Verification items for the finished model (mm, model axes). A direction names the side the tool comes from. Round coordinates to 2 decimals unless told otherwise and drop trailing zeros. Write each loop counter-clockwise with the first axis right and the second up, starting at its lowest first coordinate (ties: lowest second). Pieces come first, ordered by that corner, then holes. Notation, with made-up numbers: (62.25, 83.25) - (67.25, 83.25) arc R15 cw to (67.25, 105.25) - close; hole circle Ø11 at (12.25, -8). An arc over 180 degrees is marked (long way). Answer as a JSON object with one key per item and string values.
```python
from build123d import *

# Parameters (mm, degrees)
SKETCH1_W                        = 80
SKETCH1_H                        = 140
SKETCH1_R                        = 12.5
BOSS_EXTRUDE1_DEPTH              = 6
TAP_DRILL_FOR_M6_TAP1_D          = 5
TAP_DRILL_FOR_M6_TAP2_AT_2_COUNT = 2
TAP_DRILL_FOR_M6_TAP2_AT_2_PITCH = 32.5
TAP_DRILL_FOR_M6_TAP2_AT_3_COUNT = 2
TAP_DRILL_FOR_M6_TAP2_AT_3_PITCH = 65
TAP_DRILL_FOR_M6_TAP3_D          = 5
TAP_DRILL_FOR_M6_TAP3_DEPTH      = 26
TAP_DRILL_FOR_M6_TAP3_TIP        = 1.502151548


with BuildPart() as part:
    # Sketch1 → Boss-Extrude1 (new body, symmetric)
    with BuildSketch(Plane(origin=(0, 0, 0), x_dir=(1, 0, 0), z_dir=(0, 1, 0))):
        with Locations((0, 70)):
            Rectangle(SKETCH1_W, SKETCH1_H)
        with Locations((10, 42.5)):
            Circle(SKETCH1_R, mode=Mode.SUBTRACT)
    extrude(amount=BOSS_EXTRUDE1_DEPTH, both=True)

    # Tap Drill for M6 Tap1 (through all)
    with Locations(Plane(origin=(0, 6, 0), x_dir=(1, 0, 0), z_dir=(0, 1, 0))):
        with Locations((-25, 67.5), (25, 67.5), (25, 17.5), (-25, 17.5)):
            Hole(TAP_DRILL_FOR_M6_TAP1_D / 2)

    # Sketch9 → Tap Drill for M6 Tap2 (revolve, cut)
    with BuildSketch(Plane(origin=(32.5, 0, 0), x_dir=(0, -1, 0), z_dir=(1, 0, 0))):
        Polygon((0, 0), (0, 21.502151548), (2.5, 20), (2.5, 0), align=None)
    tap_drill_for_m6_tap2 = revolve(axis=Axis((32.5, 0, 6.35), (0, 0, -1)), mode=Mode.SUBTRACT)

    # Tap Drill for M6 Tap2 at 2: Tap Drill for M6 Tap2 ×2
    with Locations(*[(-i * TAP_DRILL_FOR_M6_TAP2_AT_2_PITCH, 0, 0) for i in range(1, TAP_DRILL_FOR_M6_TAP2_AT_2_COUNT)]):
        add(tap_drill_for_m6_tap2, mode=Mode.SUBTRACT)

    # Tap Drill for M6 Tap2 at 3: Tap Drill for M6 Tap2 ×2
    with Locations(*[(-i * TAP_DRILL_FOR_M6_TAP2_AT_3_PITCH, 0, 0) for i in range(1, TAP_DRILL_FOR_M6_TAP2_AT_3_COUNT)]):
        add(tap_drill_for_m6_tap2, mode=Mode.SUBTRACT)

    # Mirror1: Tap Drill for M6 Tap2 across plane
    add(tap_drill_for_m6_tap2.mirror(Plane(origin=(0, 0, -70), x_dir=(1, 0, 0), z_dir=(0, 0, -1))), mode=Mode.SUBTRACT)

    # Mirror1 copy 1 sketch → Mirror1 copy 1 (revolve, cut)
    with BuildSketch(Plane(origin=(0, 0, -140), x_dir=(0, -1, 0), z_dir=(1, 0, 0))):
        Polygon((0, 0), (0, -21.502151548), (2.5, -20), (2.5, 0), align=None)
    revolve(axis=Axis((0, 0, -146.35), (0, 0, -1)), mode=Mode.SUBTRACT)

    # Mirror1 copy 2 sketch → Mirror1 copy 2 (revolve, cut)
    with BuildSketch(Plane(origin=(-32.5, 0, -140), x_dir=(0, -1, 0), z_dir=(1, 0, 0))):
        Polygon((0, 0), (0, -21.502151548), (2.5, -20), (2.5, 0), align=None)
    revolve(axis=Axis((-32.5, 0, -146.35), (0, 0, -1)), mode=Mode.SUBTRACT)

    # Tap Drill for M6 Tap3
    with Locations(Plane.ZY.offset(40)):
        with Locations((-113, 0), (-86, 0), (-56, 0), (-29, 0)):
            Hole(TAP_DRILL_FOR_M6_TAP3_D / 2, depth=TAP_DRILL_FOR_M6_TAP3_DEPTH)
            with Locations((0, 0, -(TAP_DRILL_FOR_M6_TAP3_DEPTH + TAP_DRILL_FOR_M6_TAP3_TIP / 2))):  # 118° drill point
                Cone(0, TAP_DRILL_FOR_M6_TAP3_D / 2, TAP_DRILL_FOR_M6_TAP3_TIP, mode=Mode.SUBTRACT)


solid = part.part
```
Q1. Section check C-C, the plane x = 12. Record the cut outline in (y, z), then the cut area to 3 significant figures.
Geometry check:
{"outline": "(-6, -140) - (6, -140) - (6, -54.84) - (-6, -54.84) - close; (-6, -30.16) - (6, -30.16) - (6, 0) - (-6, 0) - close", "area": "1,380 mm2"}
Q2. Section check A-A, the plane x = -25. Record the cut outline in (y, z), then the cut area to 3 significant figures.
Geometry check:
{"outline": "(-6, -140) - (6, -140) - (6, -70) - (-6, -70) - close; (-6, -65) - (6, -65) - (6, -20) - (-6, -20) - close; (-6, -15) - (6, -15) - (6, 0) - (-6, 0) - close; hole circle Ø5 at (0, -113); hole circle Ø5 at (0, -86); hole circle Ø5 at (0, -56); hole circle Ø5 at (0, -29)", "area": "1,480 mm2"}
Q3. Gauge pin test, flat ends, axial feed: P1, Ø4, axis at x = -25, z = -67.5, coming from the +Y side; P2, Ø4.5, axis at y = 0, z = -86, coming from the -X side; P3, Ø4, axis at x = 32.5, y = 0, coming from the +Z side. Record the tip position at first contact, or that the pin passes through.
Geometry check:
{"P1": "passes through", "P2": "stops at x = -13.85", "P3": "stops at z = -20.3"}
Q4. Release check for a two-part mould opening along Z. For faces 1 (the flat face through (-1, 3, 0)), 2 (the cylindrical face through (-35, 0, -10)), 3 (the cylindrical face through (-23, 0, -19)) record: released by +Z, released by -Z, zero draft, split by the parting line, or undercut.
Geometry check:
{"face 1": "released by +Z", "face 2": "zero draft", "face 3": "undercut"}
Q5. Section check B-B, the plane z = -128.5. Record the cut outline in (x, y), then the cut area to 3 significant figures.
Geometry check:
{"outline": "(-40, -6) - (40, -6) - (40, 6) - (-40, 6) - close; hole circle Ø5 at (-32.5, 0); hole circle Ø5 at (0, 0); hole circle Ø5 at (32.5, 0)", "area": "901 mm2"}
Q6. Set-up check for faces 4 (the cylindrical face through (-26.8, 0.1, -26.5)), 5 (the cylindrical face through (30, 0, -130)), 6 (the cylindrical face through (2.44, 0.54, -9.86)): record each of +Z, -Z, +X, -X, +Y, -Y from which the full face is reachable in a straight line by a thin tool's end or side.
Geometry check:
{"face 4": "-X", "face 5": "-Z", "face 6": "+Z"}
Q7. Material ranges on line 1 along Z through (x, y) = (-25, 3.25); line 2 along X through (y, z) = (0, -130.5); line 3 along Z through (x, y) = (-14, 0.25), recorded low to high. Write a range as [from, to].
Geometry check:
{"line 1": "z = [-140, -70], [-65, -20], [-15, 0]", "line 2": "x = [-40, -35], [-30, -2.5], [2.5, 30], [35, 40]", "line 3": "z = [-140, -115.49], [-110.51, -88.49], [-83.51, -58.49], [-53.51, -31.49], [-26.51, 0]"}
